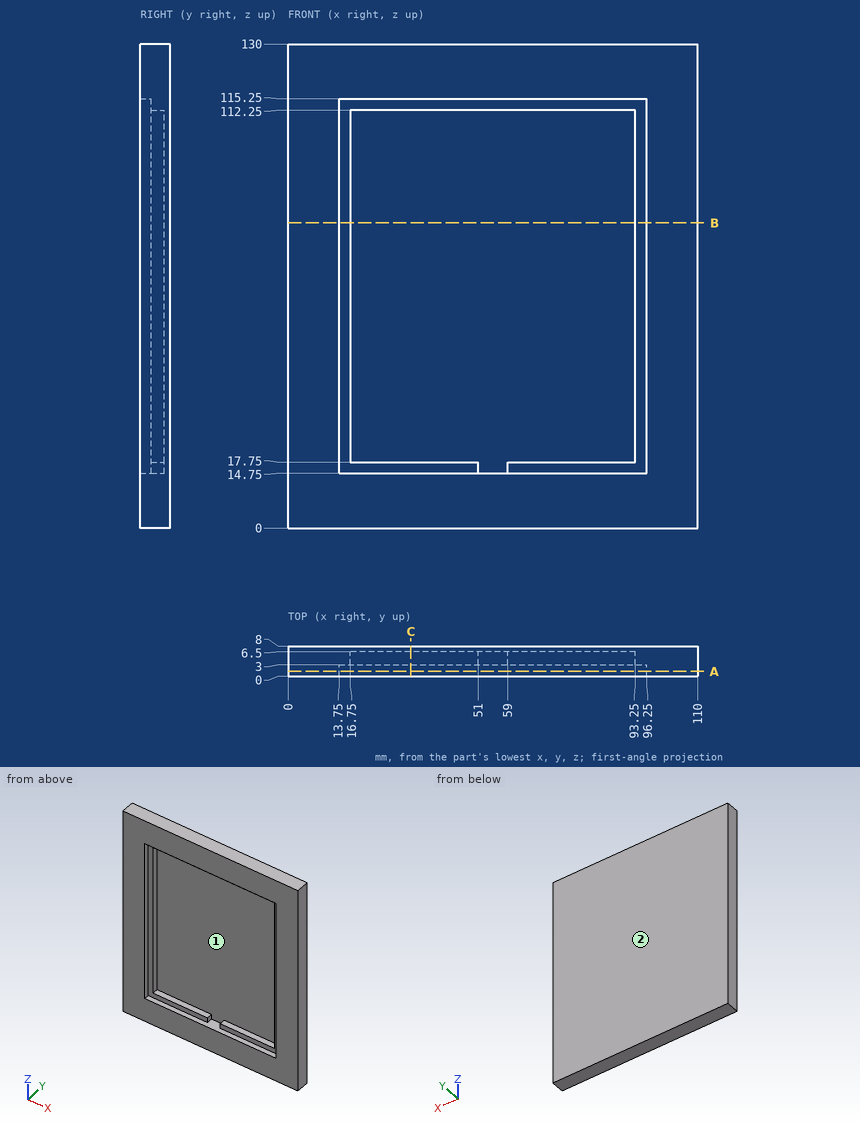
Study the drawing (mm; zero at the part's minimum x, y, z) and answer. Give positions to 0.01 mm unless a question says otherwise; leave off trailing zeros. Order: outer loops, then holes, each group sorted by start corner. A loop starts at its lowest first (then second) coordinate and runs counter-clockwise, first axis right, second up. Notation, with made-up numbers: M -4.75,-12 L 12.25,-12 A27 cw 12.25,15 Z; hole C 9,47.25 d7. An arc over 180 degrees is marked long. Put each result on its own line as item: value. Start each with the question number.
Item 1: The part is cut by section A-A, the plane y = 1.25. Determine the outline of the cut face in (x, z).
Item 2: The part is cut by section B-B, the plane z = 82. Determine the outline of the cut face in (x, y), and give its area (3 significant figures).
Item 3: Flat-ended cylindrical pins translate along their axes: P1, Ø1, axis at y = 3, z = 26.5, coming from the -X side; P2, Ø6, axis at x = 38, z = 93, coming from the -Y side. Find the tip coordinate at first contact, or state that the pin passes through.
Item 4: The part is cut by section C-C, the plane x = 33. Determine the outline of the cut face in (y, z).
Item 5: For a pull along Z with two mould halves and no side action, classify the marked faces 1 and 2 as +Z half, -Z half, draft (parallel to the pull), parting line (faces both ways), or undercut.
Item 6: Find the intervals of material crossed by line 1 along Z through (x, y) = (92, 6); line 2 along Z through (x, y) = (21, 2.25); line 3 along X through (y, z) = (5.25, 33), in increasing order.
Answer key:
1. outline: M 0,0 L 110,0 L 110,130 L 0,130 Z; hole M 13.75,14.75 L 96.25,14.75 L 96.25,115.25 L 13.75,115.25 Z
2. outline: M 0,0 L 13.75,0 L 13.75,3 L 16.75,3 L 16.75,6.5 L 93.25,6.5 L 93.25,3 L 96.25,3 L 96.25,0 L 110,0 L 110,8 L 0,8 Z
2. area: 365 mm²
3. P1: stops at x = 0
3. P2: stops at y = 6.5
4. outline: M 0,0 L 8,0 L 8,130 L 0,130 L 0,115.25 L 3,115.25 L 3,112.25 L 6.5,112.25 L 6.5,17.75 L 3,17.75 L 3,14.75 L 0,14.75 Z
5. face 1: undercut
5. face 2: draft
6. line 1: z = 0 to 17.75, 112.25 to 130
6. line 2: z = 0 to 14.75, 115.25 to 130
6. line 3: x = 0 to 16.75, 93.25 to 110
